Print and shaded views of the part. All mm, measured from the part's lowest x, y and z. Round coordinates to 2 decimals unless told otherwise and drop trailing zeros. Order: outer loops, then holes, each group sorted by start corner. A loop starts at its lowest first (then second) coordinate and runs counter-clockwise, first axis right, second up. Notation, with made-up numbers: M 36,41.5 L 40,41.5 A33 cw 40,80.5 Z; hole C -12.5,42.5 d3. An arc over 180 degrees is marked long. Use CSV: the item, a comma, the result in double quotes.
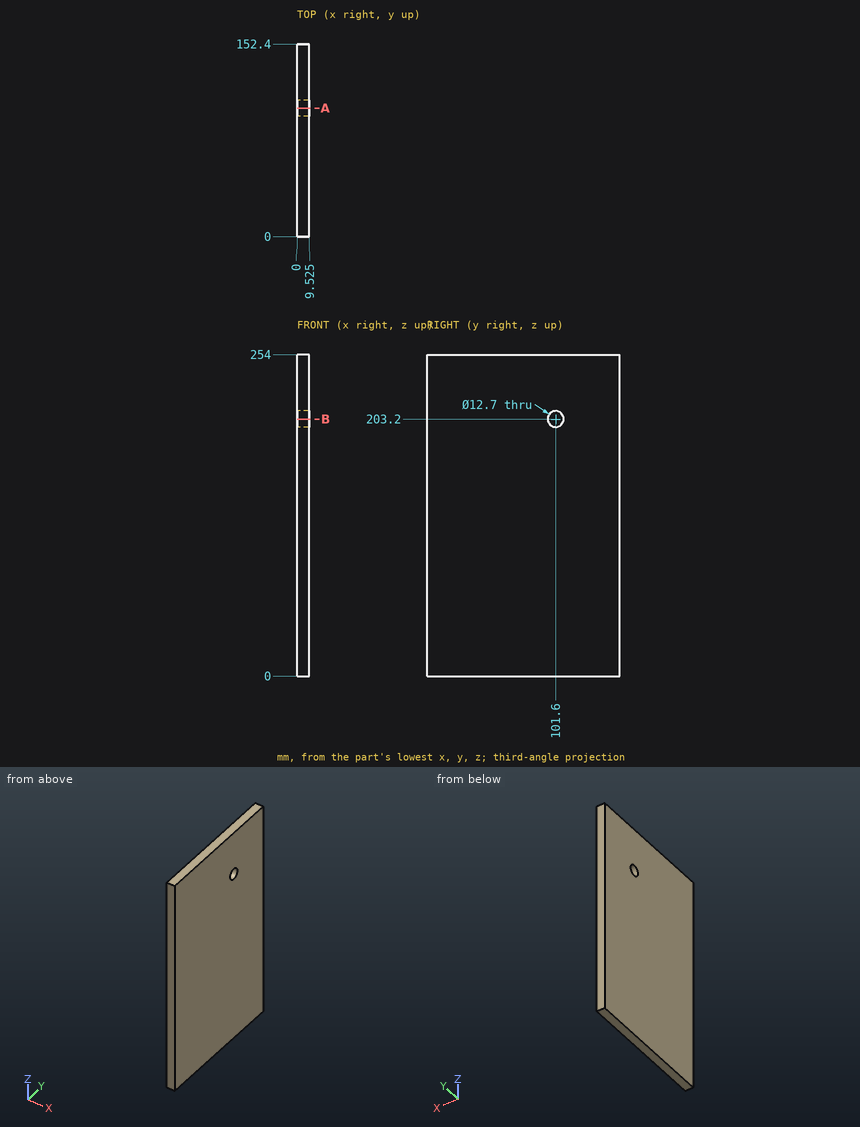
(1) Wall check: line 1 (Z direction, x = 5, y = 101.6); line 2 (Z direction, x = 8.25, y = 103.5). Give the ranges that are in metal, low to high. Write a range as from..to.
Answer block:
line 1,"z = 0..196.85, 209.55..254"
line 2,"z = 0..197.14, 209.26..254"
(2) Cut at A-A, the plane y = 101.6. Give the cut face in (x, z) (3 decimals), and give its area (3 significant figures).
Answer block:
outline,"M 0,0 L 9.525,0 L 9.525,196.85 L 0,196.85 Z; M 0,209.55 L 9.525,209.55 L 9.525,254 L 0,254 Z"
area,"2,300 mm²"
(3) Cut at B-B, the plane z = 203.2. Give the cut face in (x, y) (3 decimals).
Answer block:
outline,"M 0,0 L 9.525,0 L 9.525,95.25 L 0,95.25 Z; M 0,107.95 L 9.525,107.95 L 9.525,152.4 L 0,152.4 Z"
